from build123d import *

# Parameters (mm, degrees)
SKETCH1_R           = 2.8
BOSS_EXTRUDE1_DEPTH = 5
CUT_EXTRUDE1_REACH  = 80.329
CUT_EXTRUDE2_DEPTH  = 3
CUT_EXTRUDE3_REACH  = 59.217
SKETCH6_R           = 1.75


with BuildPart() as part:
    # Sketch1 → Boss-Extrude1 (new body)
    with BuildSketch(Plane(origin=(0, 0, 0), x_dir=(1, 0, 0), z_dir=(0, 1, 0))):
        Polygon((-40.303943114, 15.555205773), (-15.555205773, 40.303943114), (4.694794227, 40.303943114), (24.042773974, 20.955963368), (24.042773974, 0.705963368), (-0.705963368, -24.042773974), (-20.955963368, -24.042773974), (-40.303943114, -4.694794227), align=None)
        with Locations(Location((-11.666118476, -16.618152771, 0), (0, 0, 270))):
            Circle(SKETCH1_R, mode=Mode.SUBTRACT)
        with Locations(Location((16.618152771, 11.666118476, 0), (0, 0, 270))):
            Circle(SKETCH1_R, mode=Mode.SUBTRACT)
        with Locations(Location((-4.595050664, 32.879321912, 0), (0, 0, 270))):
            Circle(SKETCH1_R, mode=Mode.SUBTRACT)
        with Locations(Location((-32.879321912, 4.595050664, 0), (0, 0, 270))):
            Circle(SKETCH1_R, mode=Mode.SUBTRACT)
    extrude(amount=BOSS_EXTRUDE1_DEPTH)

    # Sketch4 → Cut-Extrude1 (cut, up to next)
    with BuildSketch(Plane(origin=(22.499368671, 0, -22.499368671), x_dir=(-0.7071067811865465, 0, -0.7071067811865487), z_dir=(0.7071067811865487, 0, -0.7071067811865465)), mode=Mode.PRIVATE) as cut_extrude1_sk1:
        with BuildLine():
            Line((13.998382969, 5), (8.998382969, 5))
            ThreePointArc((8.998382969, 5), (11.498382969, 2.5), (13.998382969, 5))
        make_face()
    cut_extrude1_tool1 = extrude(cut_extrude1_sk1.sketch, amount=-CUT_EXTRUDE1_REACH, mode=Mode.PRIVATE) & part.part
    add(cut_extrude1_tool1.solids().sort_by_distance((14.368784, 3.938967, -30.629953))[0], mode=Mode.SUBTRACT)

    # Sketch5 → Cut-Extrude2 (cut)
    with BuildSketch(Plane(origin=(0, 5, 0), x_dir=(1, 0, 0), z_dir=(0, 1, 0))):
        Polygon((-16.586947728, 21.240978239), (-19.765709682, 22.092724938), (-22.092724938, 19.765709682), (-21.240978239, 16.586947728), (-18.062216285, 15.735201029), (-15.735201029, 18.062216285), align=None)
        Polygon((4.979809098, -0.325778587), (1.801047144, 0.525968112), (-0.525968112, -1.801047144), (0.325778587, -4.979809098), (3.504540541, -5.831555797), (5.831555797, -3.504540541), align=None)
    extrude(amount=-CUT_EXTRUDE2_DEPTH, mode=Mode.SUBTRACT)

    # Sketch6 → Cut-Extrude3 (cut, up to next)
    with BuildSketch(Plane(origin=(0, 5, 0), x_dir=(1, 0, 0), z_dir=(0, 1, 0)), mode=Mode.PRIVATE) as cut_extrude3_sk1:
        with Locations(Location((-18.913962984, 18.913962984, 0), (0, 0, 270))):
            Circle(SKETCH6_R)
    cut_extrude3_tool1 = extrude(cut_extrude3_sk1.sketch, amount=-CUT_EXTRUDE3_REACH, mode=Mode.PRIVATE) & part.part
    # Sketch6 → Cut-Extrude3 (cut, up to next)
    with BuildSketch(Plane(origin=(0, 5, 0), x_dir=(1, 0, 0), z_dir=(0, 1, 0)), mode=Mode.PRIVATE) as cut_extrude3_sk2:
        with Locations(Location((2.652793843, -2.652793843, 0), (0, 0, 270))):
            Circle(SKETCH6_R)
    cut_extrude3_tool2 = extrude(cut_extrude3_sk2.sketch, amount=-CUT_EXTRUDE3_REACH, mode=Mode.PRIVATE) & part.part
    add(cut_extrude3_tool1.solids().sort_by_distance((-18.913963, 5, -18.913963))[0], mode=Mode.SUBTRACT)
    add(cut_extrude3_tool2.solids().sort_by_distance((2.652794, 5, 2.652794))[0], mode=Mode.SUBTRACT)


solid = part.part
Verification items for the finished model (mm, model axes). A direction names the side the tool comes from. Coordinates: 2 decimals unless noted, no trailing zeros. Order: outer loops, then holes, each group sorted by start corner. A loop starts at its lowest first (then second) coordinate and runs counter-clockwise, first axis right, second up. Notation, with made-up numbers: M 21,-35.75 L 25,-35.75 A25 ccw 25,-20.75 Z; hole C 74,78 d6. An arc over 180 degrees is marked long. Write each question's results on one line, items separated by ' | '.
1) Gauge pin test, flat ends, axial feed: pin 1 Ø2 at (x, z) = (2.65, 2.65) entering from -Y; pin 2 Ø3 at (x, y) = (-24.5, 2) entering from +Z. Record the tip position at first contact, or that the pin passes through.
Solved:
pin 1: passes through | pin 2: stops at z = 22
2) Release check for a two-part mould opening along X. For faces 1 (the face through (-30, 2, 15)), 2 (the face through (3.413, 3.521, -0.094)), 3 (the face through (11.842, 2.465, 11.495)) record: pulls with the +X half, pulls with the -X half, needs draft (parallel to the pull), parting line crosses it, or undercut.
Solved:
face 1: pulls with the -X half | face 2: undercut | face 3: pulls with the +X half
3) Access from +Z, -Z, +X, -X, +Y, -Y to the whole of each face (thin tool, end or side, straight path). Record for faces 4 (the face through (-10.83, 2.46, 19.29)), 5 (the face through (-18.15, 3.52, -21.66)).
Solved:
face 4: +Y, -Y | face 5: +Y
4) Scan lines: line 1 along Z through (x, y) = (-13, 2.1); line 2 along Z through (x, y) = (3.5, 1.55); line 3 along Z through (x, y) = (-17, 4.7). Record each from-to range of solid material in increasing order. Write a range as [from, to].
Solved:
line 1: z = [-40.3, 14.16], [19.08, 24.04] | line 2: z = [-40.3, 1.12], [4.18, 19.84] | line 3: z = [-38.86, -21.35], [-16.8, -2.77], [4.25, 24.04]
5) Section check A-A on y = 3.8. Record the cut outline in (x, z), plus the area to 3 significant figures.
Solved:
outline: M -40.3,-15.56 L -15.56,-40.3 L 4.69,-40.3 L 12.82,-32.18 L -32.18,12.82 L -40.3,4.69 Z; M -29.08,15.92 L 15.92,-29.08 L 24.04,-20.96 L 24.04,-0.71 L -0.71,24.04 L -20.96,24.04 Z; hole C -32.88,-4.6 d5.6; hole M -22.09,-19.77 L -19.77,-22.09 L -16.59,-21.24 L -15.74,-18.06 L -18.06,-15.74 L -21.24,-16.59 Z; hole C -11.67,16.62 d5.6; hole C -4.6,-32.88 d5.6; hole M -0.53,1.8 L 1.8,-0.53 L 4.98,0.33 L 5.83,3.5 L 3.5,5.83 L 0.33,4.98 Z; hole C 16.62,-11.67 d5.6 | area: 2,720 mm²
